Read the model definition and answer for the solid it produces. Units are mm, in the model's axes. Face numbers are marked on the shaded views. A direction names the side the tool comes from. Round coordinates to 2 decimals unless told otherwise and drop trailing zeros. Write each loop counter-clockwise with the first axis right and the second up, starting at its lowest first coordinate (ties: lowest second). Pieces come first, ordered by that corner, then holes. Notation, with made-up numbers: (-31, -7.5) -> (5, -7.5) arc R22 ccw to (5, 31.5) -> close; hole circle Ø6 at (88, 24). An arc over 180 degrees is marked (long way). Return JSON: item names as keys, results as strings. Group by question number.
(1) Straight lines are drawn through the part: line 1 (X direction, y = -12, z = 11); line 2 (Y direction, x = 30, z = 17); line 3 (Y direction, x = 7, z = 6). For each, find the intervals that lie inside material, in ascending order.
(2) For the marked faces 4 and 5, determine the directions among +Z, -Z, +X, -X, +Y, -Y from which every point of the face is accessible in a straight line to the end or side of a thin tool.
(3) A cutting plane is placed at D-D on x = 18. Give the vertices of the cut face in (y, z).
(4) A cutting plane is placed at B-B on x = 30. Give the vertices of the cut face in (y, z).
(5) The mould has two halves that part along X. Classify the marked faces 1, 2 and 3: released by +X, released by -X, zero draft, split by the parting line, or undercut.
(6) A cutting plane is placed at C-C on z = 17. Give the vertices of the cut face in (x, y), then the cut area to 3 significant figures.
(7) A cutting plane is placed at A-A on y = -12.5. Give the vertices of the cut face in (x, z), then the cut area to 3 significant figures.
(8) Given pin 1 (8 mm diameter, centred on x = 11.5, z = 32.5, fed in from -Y); pin 2 (17 mm diameter, centred on x = 30, y = -12.5, fed in from +Z); pin 3 (3 mm diameter, centred on y = -14.5, z = 25, fed in from -X), each flat-ended and moving along its own axis, determine where each tip first touches the part or whether it passes through.
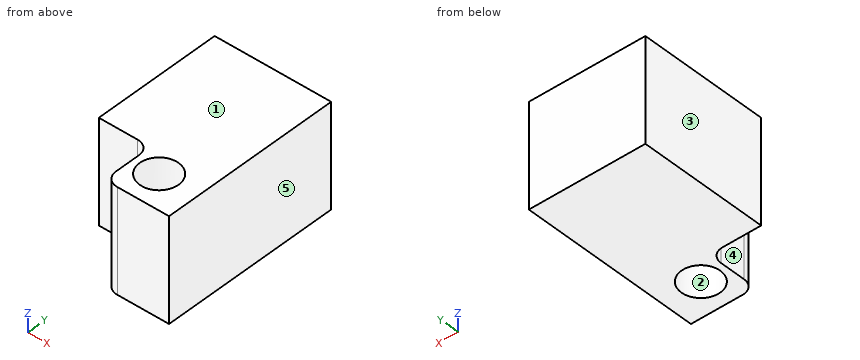
```python
from build123d import *

# Parameters (mm, degrees)
F0_R     = 7.5
F1_DEPTH = 40


# Not quite as in the source:
# - a feature names something its author has since deleted; it is built from what else it names


with BuildPart() as f1:
    # F0 (on Top) → F1 (new body)
    with BuildSketch(Plane.XY):
        with BuildLine():
            Line((40, 0), (0, 0))
            Line((0, 0), (0, -5))
            Line((0, -5), (15, -5))
            ThreePointArc((15, -5), (18.5355339059, -6.4644660941), (20, -10))
            Line((20, -10), (20, -20))
            ThreePointArc((20, -20), (21.4644660941, -23.5355339059), (25, -25))
            Line((25, -25), (35, -25))
            Line((35, -25), (45, -25))
            Line((45, -25), (45, -19.1631559283))
            Line((45, -19.1631559283), (45, 0))
            Line((45, 0), (40, 0))
        make_face()
        with Locations((30, -12.5)):
            Circle(F0_R, mode=Mode.SUBTRACT)
        Polygon((0, 45), (0, 0), (40, 0), (45, 0), (45, 45), align=None)
    extrude(amount=F1_DEPTH)


solid = f1.part
```
Checks:
{
 "1": {"line 1": "x = 20 to 22.52, 37.48 to 45", "line 2": "y = -25 to -20, -5 to 45", "line 3": "y = -5 to 45"},
 "2": {"face 4": "+Z, -Z, -X, -Y", "face 5": "+Z, -Z, +X, +Y, -Y"},
 "3": {"outline": "(-6, 0) -> (45, 0) -> (45, 40) -> (-6, 40) -> close"},
 "4": {"outline": "(-25, 0) -> (-20, 0) -> (-20, 40) -> (-25, 40) -> close; (-5, 0) -> (45, 0) -> (45, 40) -> (-5, 40) -> close"},
 "5": {"face 1": "zero draft", "face 2": "undercut", "face 3": "released by -X"},
 "6": {"outline": "(0, -5) -> (15, -5) arc R5 cw to (20, -10) -> (20, -20) arc R5 ccw to (25, -25) -> (45, -25) -> (45, 45) -> (0, 45) -> close; hole circle Ø15 at (30, -12.5)", "area": "2,570 mm^2"},
 "7": {"outline": "(20, 0) -> (22.5, 0) -> (22.5, 40) -> (20, 40) -> close; (37.5, 0) -> (45, 0) -> (45, 40) -> (37.5, 40) -> close", "area": "400 mm^2"},
 "8": {"pin 1": "stops at y = -5.03", "pin 2": "stops at z = 40", "pin 3": "stops at x = 20"}
}
